Check sheet for the modelled part. Datum: model origin and axes. Units: mm. Face numbers are marked on the shaded views. Give positions to 0.01 mm unless a question says otherwise; leave off trailing zeros. Loops run counter-clockwise (first coordinate to the right, second up) from the corner with the lowest first, then second, coordinate; pieces in that order, holes last. Notation, with made-up numbers: (67, 64) - (89, 64) arc R18 ccw to (89, 86) - close; hole circle Ø4 at (-34, 66). An arc over 180 degrees is marked (long way). Use one line per item in the form item = value.
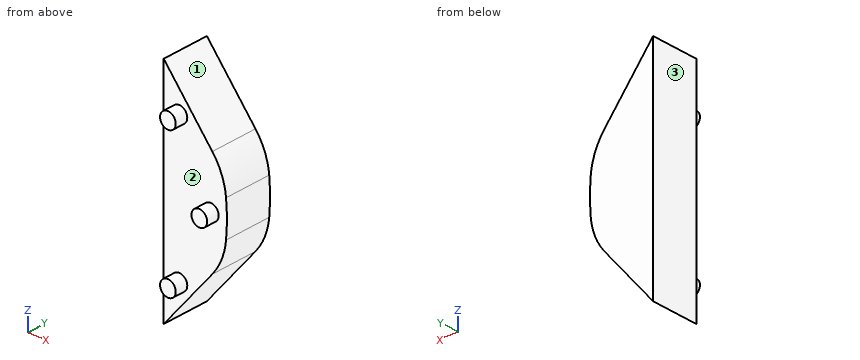
from build123d import *

# Parameters (mm, degrees)
BOSS_EXTRUDE2_DEPTH = 38.1
SKETCH4_R           = 6.35
BOSS_EXTRUDE3_DEPTH = 10.16
CUT_EXTRUDE1_DEPTH  = 72.136
FILLET1_R           = 50.8


with BuildPart() as part:
    # Sketch3 → Boss-Extrude2 (new body)
    with BuildSketch(Plane(origin=(0, 0, 0), x_dir=(1, 0, 0), z_dir=(0, 1, 0))):
        with BuildLine():
            Line((0, 90.272622301), (0, -90.272622301))
            add(Edge.make_bspline(
                [(0, -90.272622301), (51.063722035, -90.272622301), (51.063722035, 0), (51.063722035, 90.272622301), (0, 90.272622301)],
                knots=[3.141592654, 3.141592654, 3.141592654, 4.71238898, 4.71238898, 6.283185307, 6.283185307, 6.283185307], degree=2, weights=[1, 0.707106781, 1, 0.707106781, 1]))
        make_face()
    extrude(amount=BOSS_EXTRUDE2_DEPTH)

    # Sketch4 → Boss-Extrude3 (add)
    with BuildSketch(Plane(origin=(0, 0, 0), x_dir=(-1, 0, 0), z_dir=(0, -1, 0))):
        with Locations(Location((-12.7, -57.15, 0), (0, 0, 270))):
            Circle(SKETCH4_R)
        with Locations(Location((-12.7, 57.15, 0), (0, 0, 270))):
            Circle(SKETCH4_R)
        with Locations(Location((-38.1, 0, 0), (0, 0, 270))):
            Circle(SKETCH4_R)
    extrude(amount=BOSS_EXTRUDE3_DEPTH)

    # Sketch5 → Cut-Extrude1 (cut)
    with BuildSketch(Plane(origin=(0, 0, 0), x_dir=(-1, 0, 0), z_dir=(0, -1, 0))):
        Polygon((0, -90.272622301), (-47.948224184, -31.049250245), (-73.055798017, -65.580157533), (-28.861670947, -122.242067224), align=None)
        Polygon((0, 90.272622301), (-47.948224184, 31.049250245), (-64.283944167, 60.660936273), (-1.502105519, 110.713212963), align=None)
    extrude(amount=-CUT_EXTRUDE1_DEPTH, mode=Mode.SUBTRACT)

    # Fillet1
    fillet1_edges = [part.edges().sort_by_distance(p)[0] for p in [
        (47.948224184, 19.05, -31.049250245),
        (47.948224184, 19.05, 31.049250245),
    ]]
    fillet(fillet1_edges, radius=FILLET1_R)


solid = part.part
Item 1: Gauge pin test, flat ends, axial feed: P1, Ø8, axis at y = 4, z = 39, coming from the +X side; P2, Ø5, axis at y = 11, z = -6.5, coming from the +X side; P3, Ø2, axis at x = 7, z = 71, coming from the -Y side. Record the tip position at first contact, or that the pin passes through.
Answer block:
P1 = 43.91
P2 = 51.01
P3 = 0
Item 2: Section check B-B on x = 15. Record the boundary of the cut face in (y, z), then the cut area to 3 significant figures.
Answer block:
outline = (-10.16, -63.07) - (0, -63.07) - (0, -71.75) - (38.1, -71.75) - (38.1, 71.75) - (0, 71.75) - (0, 63.07) - (-10.16, 63.07) - (-10.16, 51.23) - (0, 51.23) - (0, -51.23) - (-10.16, -51.23) - close
area = 5,710 mm2
Item 3: Section check C-C on z = -47. Record the boundary of the cut face in (x, y).
Answer block:
outline = (0, 0) - (35.03, 0) - (35.03, 38.1) - (0, 38.1) - close
Item 4: Section check D-D on x = 24.5. Record the boundary of the cut face in (y, z).
Answer block:
outline = (0, -60.01) - (38.1, -60.01) - (38.1, 60.01) - (0, 60.01) - close
Item 5: Thickness scan on L1, parallel to Y at x = 4, z = 20.5; L2, parallel to X at y = 12, z = 38.5; L3, parallel to X at y = 0.5, z = -34. Record the ranges inside material, lowest first.
Answer block:
L1 = 0 to 38.1
L2 = 0 to 41.71
L3 = 0 to 44.47
Item 6: Mould release check, pull along Z, two halves, no side actions. Record for the marked faces 1, 2 and 3: released by +Z, released by -Z, zero draft, split by the parting line, or undercut.
Answer block:
face_1 = released by +Z
face_2 = undercut
face_3 = zero draft
Item 7: Section check A-A on z = 52.5. Record the boundary of the cut face in (x, y).
Answer block:
outline = (0, 0) - (8.38, 0) - (8.38, -10.16) - (17.02, -10.16) - (17.02, 0) - (30.58, 0) - (30.58, 38.1) - (0, 38.1) - close
